Verification items for the finished model (mm, model axes). A direction names the side the tool comes from. Coordinates: 2 decimals unless noted, no trailing zeros. Order: outer loops, then holes, each group sorted by start corner. A loop starts at its lowest first (then second) coordinate and runs counter-clockwise, first axis right, second up. Notation, with made-up numbers: (-9.75, 71.5) -> (44.25, 71.5) arc R21 cw to (44.25, 99.5) -> close; hole circle Ø11 at (-26, 43.25). An arc over 180 degrees is marked (long way). Write each question's results on one line, items separated by ' | '. Start each with the question number.
(1) Cross-section at A-A on z = 28.5. Enter the section's corners in (x, y), and give its area (3 significant figures).
(2) Set-up check for faces 1 (the flat face through (65, 4, 11)), 2 (the flat face through (1, 63.75, 50)): record each of +Z, -Z, +X, -X, +Y, -Y from which the full face is reachable in a straight line by a thin tool's end or side.
(3) Thickness scan on probe 1 along Z at (x, y) = (74, 63); probe 2 along Y at (x, z) = (6.5, 24); probe 3 along Z at (x, y) = (55.5, 61). Record the ranges inside material, lowest first. Write a range as [from, to].
(4) Draft check along Z on faces 3 (the flat face through (1, 21.917, 44)), 4 (the flat face through (1, 21.917, 50)), 5 (the flat face through (65, 65, 44)). Enter one of: +Z half, -Z half, draft (parallel to the pull), parting line (faces both ways), or undercut.
(5) Cross-section at B-B on x = 34.5. Enter the section's corners in (y, z), and give its area (3 significant figures).
(6) Go/stop test with flat-tipped pins: pin 1 (1.2 mm diameter, centred on x = 1.5, y = 29.5, fed in from -Z); pin 2 (5 mm diameter, centred on y = 41.5, z = 15, fed in from +X); pin 3 (10 mm diameter, centred on x = 16, y = 56.5, fed in from +Z). Record where each tip stops, or that it passes through.
```python
from build123d import *

# Parameters (mm, degrees)
F1_DEPTH = 130
F2_W     = 14
F2_H     = 12
F2_W_2   = 12.5
F2_H_2   = 3.5
F3_DEPTH = 2.5


with BuildPart() as f1:
    # F0 (on Right) → F1 (new body)
    with BuildSketch(Plane.YZ):
        Polygon((0, 32), (0, 0), (69, 0), (69, 65), (65, 65), (65, 22), (62.5, 22), (62.5, 21), (65, 21), (65, 19), (62.5, 19), (62.5, 18), (65, 18), (65, 4), (4, 4), (4, 18), (6.5, 18), (6.5, 19), (4, 19), (4, 21), (6.5, 21), (6.5, 22), (4, 22), (4, 32), align=None)
    extrude(amount=F1_DEPTH)

    # F2 (on face) → F3 (join)
    with BuildSketch(Plane(origin=(0, 0, 0), x_dir=(0, -1, 0), z_dir=(-1, 0, 0))):
        Polygon((-4, 32), (0, 32), (0, 65), (-65, 65), (-65, 22), (-62.5, 22), (-62.5, 21), (-65, 21), (-65, 19), (-62.5, 19), (-62.5, 18), (-65, 18), (-65, 4), (-4, 4), (-4, 18), (-6.5, 18), (-6.5, 19), (-4, 19), (-4, 21), (-6.5, 21), (-6.5, 22), (-4, 22), align=None)
        with Locations((-49, 14.5)):
            Rectangle(F2_W, F2_H, mode=Mode.SUBTRACT)
        with BuildLine():
            Line((-42, 23.5), (-56, 23.5))
            ThreePointArc((-56, 23.5), (-61, 28.5), (-56, 33.5))
            Line((-56, 33.5), (-42, 33.5))
            ThreePointArc((-42, 33.5), (-37, 28.5), (-42, 23.5))
        make_face(mode=Mode.SUBTRACT)
        Polygon((-11.5, 31.5), (-7, 31.5), (-7, 21.5), (-16, 21.5), (-16, 8.5), (-26, 8.5), (-26, 21.5), (-31, 21.5), (-31, 31.5), (-26.5, 31.5), (-26.5, 33.5), (-24.5, 33.5), (-24.5, 31.5), (-13.5, 31.5), (-13.5, 33.5), (-11.5, 33.5), align=None, mode=Mode.SUBTRACT)
        with Locations((-57.5, 37.75)):
            Rectangle(F2_W_2, F2_H_2, mode=Mode.SUBTRACT)
        with Locations((-57.5, 43.75)):
            Rectangle(F2_W_2, F2_H_2, mode=Mode.SUBTRACT)
        with Locations((-42.833333, 37.75)):
            Rectangle(F2_W_2, F2_H_2, mode=Mode.SUBTRACT)
        with Locations((-42.833333, 43.75)):
            Rectangle(F2_W_2, F2_H_2, mode=Mode.SUBTRACT)
        with Locations((-57.5, 49.75)):
            Rectangle(F2_W_2, F2_H_2, mode=Mode.SUBTRACT)
        with Locations((-57.5, 55.75)):
            Rectangle(F2_W_2, F2_H_2, mode=Mode.SUBTRACT)
        with Locations((-42.833333, 49.75)):
            Rectangle(F2_W_2, F2_H_2, mode=Mode.SUBTRACT)
        with Locations((-42.833333, 55.75)):
            Rectangle(F2_W_2, F2_H_2, mode=Mode.SUBTRACT)
        with Locations((-28.166667, 37.75)):
            Rectangle(F2_W_2, F2_H_2, mode=Mode.SUBTRACT)
        with Locations((-28.166667, 43.75)):
            Rectangle(F2_W_2, F2_H_2, mode=Mode.SUBTRACT)
        with Locations((-13.5, 37.75)):
            Rectangle(F2_W_2, F2_H_2, mode=Mode.SUBTRACT)
        with Locations((-13.5, 43.75)):
            Rectangle(F2_W_2, F2_H_2, mode=Mode.SUBTRACT)
        with Locations((-28.166667, 49.75)):
            Rectangle(F2_W_2, F2_H_2, mode=Mode.SUBTRACT)
        with Locations((-28.166667, 55.75)):
            Rectangle(F2_W_2, F2_H_2, mode=Mode.SUBTRACT)
        with Locations((-13.5, 49.75)):
            Rectangle(F2_W_2, F2_H_2, mode=Mode.SUBTRACT)
        with Locations((-13.5, 55.75)):
            Rectangle(F2_W_2, F2_H_2, mode=Mode.SUBTRACT)
    extrude(amount=-F3_DEPTH)


solid = f1.part
```
Results are:
1) outline: (0, 0) -> (130, 0) -> (130, 4) -> (2.5, 4) -> (2.5, 7) -> (0, 7) -> close; (0, 31) -> (2.5, 31) -> (2.5, 37) -> (0, 37) -> close; (0, 61) -> (2.5, 61) -> (2.5, 65) -> (130, 65) -> (130, 69) -> (0, 69) -> close | area: 1,070 mm2
2) face 1: +X | face 2: +X, -X
3) probe 1: z = [0, 4], [18, 19], [21, 22] | probe 2: y = [0, 4], [65, 69] | probe 3: z = [0, 4]
4) face 3: undercut | face 4: undercut | face 5: draft
5) outline: (0, 0) -> (69, 0) -> (69, 65) -> (65, 65) -> (65, 22) -> (62.5, 22) -> (62.5, 21) -> (65, 21) -> (65, 19) -> (62.5, 19) -> (62.5, 18) -> (65, 18) -> (65, 4) -> (4, 4) -> (4, 18) -> (6.5, 18) -> (6.5, 19) -> (4, 19) -> (4, 21) -> (6.5, 21) -> (6.5, 22) -> (4, 22) -> (4, 32) -> (0, 32) -> close | area: 642 mm2
6) pin 1: stops at z = 0 | pin 2: stops at x = 2.5 | pin 3: stops at z = 4
